The figure shows three views and two pictorial views of one solid part (mm, origin at its lowest corner). Answer the questions. Give positions to 0.01 mm unless a question says otherwise; leave off trailing zeros. Loops run counter-clockwise (first coordinate to the right, second up) from the corner with the lowest first, then second, coordinate; pieces in that order, holes last. Notation, with made-up numbers: (-25, 17.5) -> (33, 17.5) arc R7 ccw to (33, 29.5) -> close; hole circle Ø11 at (-27.5, 33). An arc over 180 degrees is marked (long way). One line per item, written item: value. Start each with the question number.
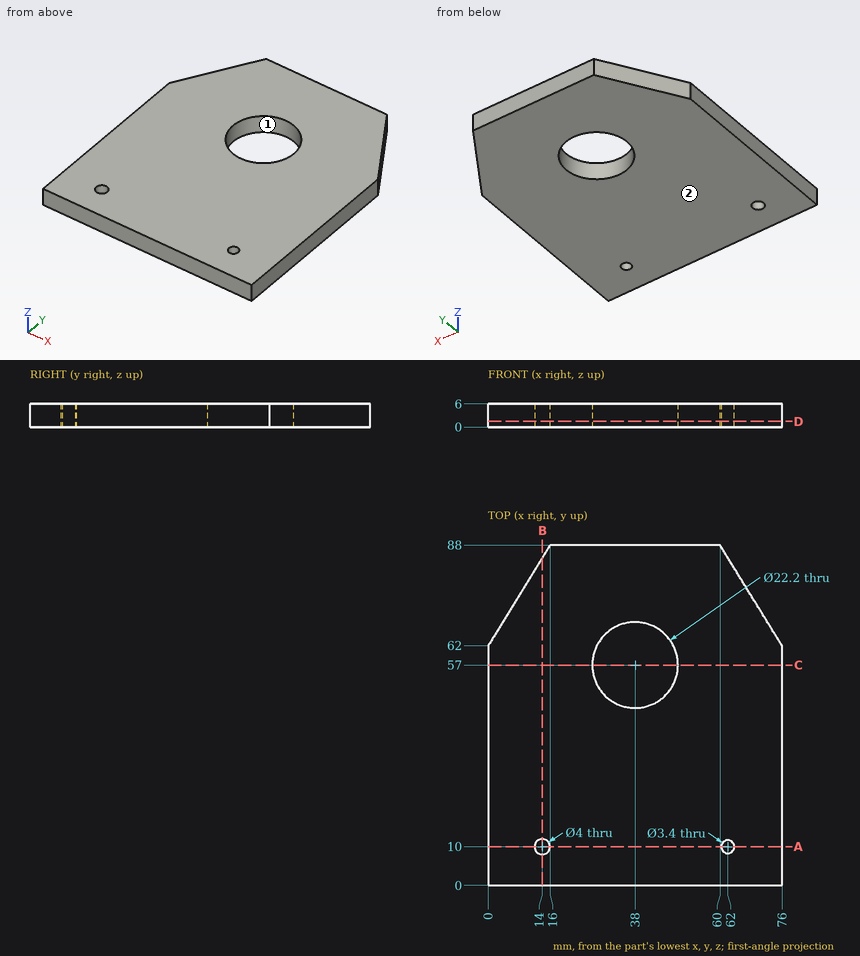
Item 1: Consider L1, parallel to Y at x = 38, z = 1.75; L2, parallel to X at y = 64.5, z = 1.65; L3, parallel to Y at x = 62, z = 3. Determine where each line is inside the solid, lowest interval first. Write a range as [from, to].
Item 2: Section A-A, the plane y = 10 is taken. Determine the outline of the cut face in (x, z), plus the area to 3 significant figures.
Item 3: Section C-C, the plane y = 57 is taken. Determine the outline of the cut face in (x, z), plus the area to 3 significant figures.
Item 4: Determine the mould class of the marked faces 1 and 2 for opening direction X: pulls with the +X half, pulls with the -X half, needs draft (parallel to the pull), parting line crosses it, or undercut.
Item 5: Section B-B, the plane x = 14 is taken. Determine the outline of the cut face in (y, z), plus the area to 4 significant figures.
Item 6: Section D-D, the plane z = 1.5 is taken. Determine the outline of the cut face in (x, y).
Computed values:
1. L1: [0, 45.9], [68.1, 88]
1. L2: [1.54, 29.82], [46.18, 74.46]
1. L3: [0, 8.3], [11.7, 84.75]
2. outline: (0, 0) -> (12, 0) -> (12, 6) -> (0, 6) -> close; (16, 0) -> (60.3, 0) -> (60.3, 6) -> (16, 6) -> close; (63.7, 0) -> (76, 0) -> (76, 6) -> (63.7, 6) -> close
2. area: 412 mm²
3. outline: (0, 0) -> (26.9, 0) -> (26.9, 6) -> (0, 6) -> close; (49.1, 0) -> (76, 0) -> (76, 6) -> (49.1, 6) -> close
3. area: 323 mm²
4. face 1: undercut
4. face 2: needs draft
5. outline: (0, 0) -> (8, 0) -> (8, 6) -> (0, 6) -> close; (12, 0) -> (84.75, 0) -> (84.75, 6) -> (12, 6) -> close
5. area: 484.5 mm²
6. outline: (0, 0) -> (76, 0) -> (76, 62) -> (60, 88) -> (16, 88) -> (0, 62) -> close; hole circle Ø4 at (14, 10); hole circle Ø22.2 at (38, 57); hole circle Ø3.4 at (62, 10)
